Here's the drawing with two shaded views (mm, measured from the low corner). I have some questions. A direction names the side the tool comes from. Give positions to 0.01 mm unless a question says otherwise; leave off trailing zeros. Write each loop counter-clockwise with the first axis right and the second up, starting at its lowest first coordinate (ties: lowest second). Pieces come first, ordered by that corner, then holes.
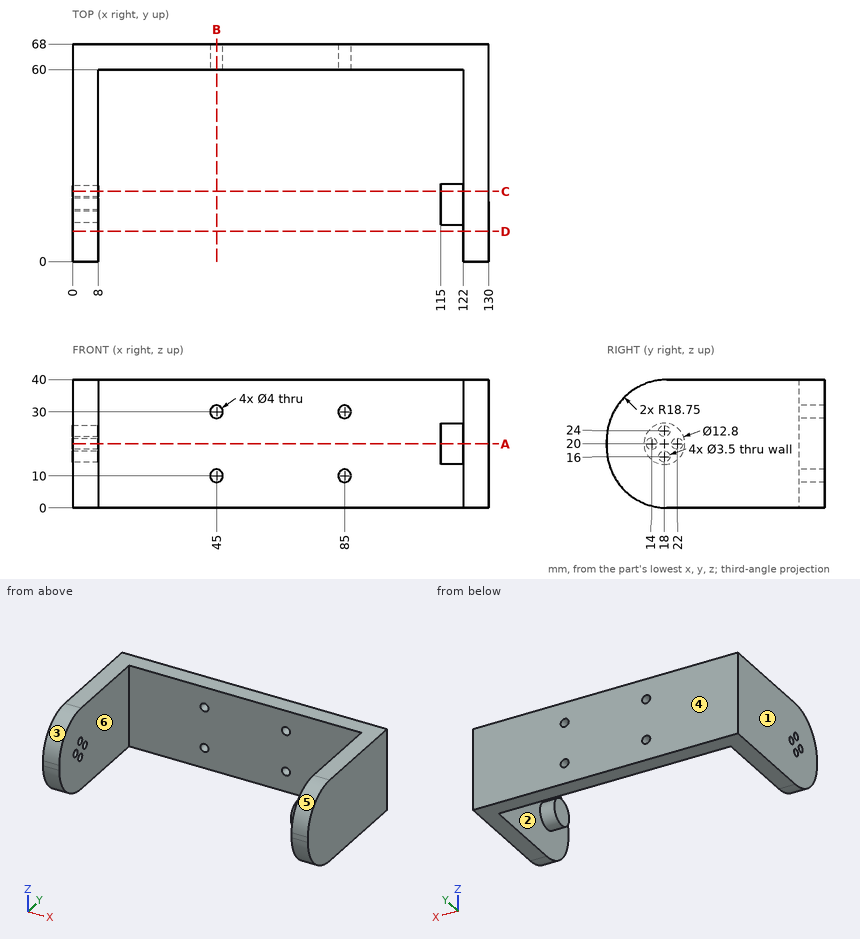
1) Suppose I cut it at B-B on x = 45. Write out the boundary of the cut face in (y, z).
Values follow:
outline: (60, 0) - (68, 0) - (68, 8) - (60, 8) - close; (60, 12) - (68, 12) - (68, 28) - (60, 28) - close; (60, 32) - (68, 32) - (68, 40) - (60, 40) - close
2) For the marked faces 5 and 6, which set-ups out of +Z, -Z, +X, -X, +Y, -Y let a thin tool reach every point of the face, with its end or its side?
Values follow:
face 5: +Z, +X, -X, -Y
face 6: +Z, -Z, -Y
3) Suppose I cut it at D-D on y = 9.5. Write out the boundary of the cut face in (x, z).
Values follow:
outline: (0, 2.44) - (8, 2.44) - (8, 37.56) - (0, 37.56) - close; (122, 2.44) - (130, 2.44) - (130, 37.56) - (122, 37.56) - close
4) Please list where these lines run through material, in increasing order: L1, parallel to Y at x = 5, z = 20; L2, parallel to Z at x = 45, y = 65.25; L3, parallel to X at y = 45, z = 29.
Values follow:
L1: y = 0 to 12.25, 15.75 to 20.25, 23.75 to 68
L2: z = 0 to 8, 12 to 28, 32 to 40
L3: x = 0 to 8, 122 to 130
5) Suppose I cut it at A-A on z = 20. Write out the boundary of the cut face in (x, y), plus the area to 3 significant figures.
Values follow:
outline: (0, 0) - (8, 0) - (8, 12.25) - (0, 12.25) - close; (0, 15.75) - (8, 15.75) - (8, 20.25) - (0, 20.25) - close; (0, 23.75) - (8, 23.75) - (8, 60) - (122, 60) - (122, 24.4) - (115, 24.4) - (115, 11.6) - (122, 11.6) - (122, 0) - (130, 0) - (130, 68) - (0, 68) - close
area: 2,030 mm2
6) Suppose I cut it at C-C on y = 22. Write out the boundary of the cut face in (x, z).
Values follow:
outline: (0, 0) - (8, 0) - (8, 18.25) - (0, 18.25) - close; (0, 21.75) - (8, 21.75) - (8, 40) - (0, 40) - close; (115, 15) - (122, 15) - (122, 0) - (130, 0) - (130, 40) - (122, 40) - (122, 25) - (115, 25) - close
7) If we mould it in two halves opening along Y, with no side actions, what happens to the marked faces 1, 2, 3 and 4? For each: +Y half, -Y half, draft (parallel to the pull), parting line (faces both ways), or undercut.
Values follow:
face 1: draft
face 2: undercut
face 3: -Y half
face 4: +Y half
8) For pin 1 Ø6.5 at (x, z) = (45, 10) entering from -Y; pin 2 Ø3 at (x, z) = (85, 10) entering from +Y, each with a flat end and sliding along its axis, tell me the tip position at first contact or that it passes through.
Values follow:
pin 1: stops at y = 60
pin 2: passes through
